Source: CAD feature listing. Evaluate the final solid. Frame: model axes, mm. A direction names the side the tool comes from. Coordinates: 2 decimals unless noted, no trailing zeros. Loops run counter-clockwise (first coordinate to the right, second up) from the corner with the lowest first, then second, coordinate; pieces in that order, holes last. Notation, with made-up numbers: M 69.5,59.5 L 87.5,59.5 A10 cw 87.5,77.5 Z; hole C -38,60 d4. An arc over 180 degrees is marked long. Write each question's results on one line, items separated by ' | '. Start each with the question number.
from build123d import *

# Parameters (mm, degrees)
BOSS_EXTRUDE2_DEPTH   = 34
SKETCH3_W             = 180.49084133
SKETCH3_H             = 138
CUT_EXTRUDE1_DEPTH    = 14
SKETCH4_R             = 11.5
SKETCH4_R_2           = 1.6
SKETCH4_R_3           = 6
CUT_EXTRUDE3_DEPTH    = 227.1769219
SKETCH5_W             = 42
SKETCH5_H             = 44
CUT_EXTRUDE4_DEPTH    = 8
M3_TAPPED_HOLE1_D     = 2.5
M3_TAPPED_HOLE1_DEPTH = 20
M3_TAPPED_HOLE1_TIP   = 0.751075774
SKETCH9_R             = 10.5
SKETCH9_R_2           = 7
CUT_EXTRUDE6_DEPTH    = 220.956813959
SKETCH10_R            = 11.5
CUT_EXTRUDE7_DEPTH    = 6
SKETCH11_R            = 13
CUT_EXTRUDE8_DEPTH    = 34
CHAMFER1_SIZE         = 6
FILLET1_R             = 10
SKETCH12_R            = 1.5
CUT_EXTRUDE9_DEPTH    = 30
SKETCH13_R            = 2.75
CUT_EXTRUDE10_DEPTH   = 3.5


with BuildPart() as part:
    # Sketch1 → Boss-Extrude2 (new body)
    with BuildSketch(Plane.XY):
        with BuildLine():
            Line((0, 0), (70, 0))
            Line((70, 0), (70, 62))
            Line((70, 62), (76, 68))
            Line((76, 68), (90, 68))
            ThreePointArc((90, 68), (97.071067812, 70.928932188), (100, 78))
            Line((100, 78), (100, 190))
            ThreePointArc((100, 190), (97.071067812, 197.071067812), (90, 200))
            Line((90, 200), (37.257365568, 200))
            ThreePointArc((37.257365568, 200), (31.383783185, 198.093270661), (27.750067173, 193.100205998))
            Line((27.750067173, 193.100205998), (-15, 62))
            Line((-15, 62), (-15, 34))
            Line((-15, 34), (0, 34))
            Line((0, 34), (0, 0))
        make_face()
    extrude(amount=BOSS_EXTRUDE2_DEPTH)

    # Sketch3 → Cut-Extrude1 (cut)
    with BuildSketch(Plane(origin=(0, 0, 0), x_dir=(-1, 0, 0), z_dir=(0, 0, -1))):
        with Locations((-9.754579335, 131)):
            Rectangle(SKETCH3_W, SKETCH3_H)
    extrude(amount=-CUT_EXTRUDE1_DEPTH, mode=Mode.SUBTRACT)

    # Sketch4 → Cut-Extrude3 (cut, through all)
    with BuildSketch(Plane.XY.offset(34)):
        with Locations((80, 134)):
            Circle(SKETCH4_R)
        with Locations((95.5, 149.5)):
            Circle(SKETCH4_R_2)
        with Locations((95.5, 118.5)):
            Circle(SKETCH4_R_2)
        with Locations((64.5, 118.5)):
            Circle(SKETCH4_R_2)
        with Locations((64.5, 149.5)):
            Circle(SKETCH4_R_2)
        with Locations((80, 174)):
            Circle(SKETCH4_R_3)
        with Locations((80, 94)):
            Circle(SKETCH4_R_3)
    extrude(amount=-CUT_EXTRUDE3_DEPTH, mode=Mode.SUBTRACT)

    # Sketch5 → Cut-Extrude4 (cut)
    with BuildSketch(Plane.XY.offset(34)):
        with Locations((79, 134)):
            Rectangle(SKETCH5_W, SKETCH5_H)
    extrude(amount=-CUT_EXTRUDE4_DEPTH, mode=Mode.SUBTRACT)

    # M3 Tapped Hole1
    with Locations(Plane(origin=(100, 0, 0), x_dir=(0, 0, -1), z_dir=(1, 0, 0))):
        with Locations((-24, 174), (-24, 94)):
            Hole(M3_TAPPED_HOLE1_D / 2, depth=M3_TAPPED_HOLE1_DEPTH)
            with Locations((0, 0, -(M3_TAPPED_HOLE1_DEPTH + M3_TAPPED_HOLE1_TIP / 2))):  # 118° drill point
                Cone(0, M3_TAPPED_HOLE1_D / 2, M3_TAPPED_HOLE1_TIP, mode=Mode.SUBTRACT)

    # Sketch9 → Cut-Extrude6 (cut, through all)
    with BuildSketch(Plane(origin=(70, 0, 0), x_dir=(0, 0, -1), z_dir=(1, 0, 0))):
        with Locations((-17, 47)):
            Circle(SKETCH9_R)
        with Locations((-17, 18)):
            Circle(SKETCH9_R_2)
    extrude(amount=-CUT_EXTRUDE6_DEPTH, mode=Mode.SUBTRACT)

    # Sketch10 → Cut-Extrude7 (cut)
    with BuildSketch(Plane.ZY):
        with Locations(Location((17, 18, 0), (0, 0, 270))):
            Circle(SKETCH10_R)
    extrude(amount=-CUT_EXTRUDE7_DEPTH, mode=Mode.SUBTRACT)

    # Sketch11 → Cut-Extrude8 (cut)
    with BuildSketch(Plane(origin=(70, 0, 0), x_dir=(0, 0, -1), z_dir=(1, 0, 0))):
        with Locations((-17, 18)):
            Circle(SKETCH11_R)
    extrude(amount=-CUT_EXTRUDE8_DEPTH, mode=Mode.SUBTRACT)

    # Chamfer1
    chamfer1_edges = [part.edges().sort_by_distance(p)[0] for p in [
        (27.5, 62, 0),
        (27.5, 62, 14),
    ]]
    chamfer(chamfer1_edges, length=CHAMFER1_SIZE)

    # Fillet1
    fillet1_edges = [part.edges().sort_by_distance(p)[0] for p in [
        (35, 0, 0),
        (35, 0, 34),
    ]]
    fillet(fillet1_edges, radius=FILLET1_R)

    # Sketch12 → Cut-Extrude9 (cut)
    with BuildSketch(Plane.ZY.offset(-6)):
        with Locations((17, 26)):
            Circle(SKETCH12_R)
        with Locations((25, 18)):
            Circle(SKETCH12_R)
        with Locations((17, 10)):
            Circle(SKETCH12_R)
        with Locations((9, 18)):
            Circle(SKETCH12_R)
    extrude(amount=-CUT_EXTRUDE9_DEPTH, mode=Mode.SUBTRACT)

    # Sketch13 → Cut-Extrude10 (cut)
    with BuildSketch(Plane(origin=(0, 0, 14), x_dir=(-1, 0, 0), z_dir=(0, 0, -1))):
        with Locations((-95.5, 149.5)):
            Circle(SKETCH13_R)
        with Locations((-64.5, 149.5)):
            Circle(SKETCH13_R)
        with Locations((-64.5, 118.5)):
            Circle(SKETCH13_R)
        with Locations((-95.5, 118.5)):
            Circle(SKETCH13_R)
    extrude(amount=-CUT_EXTRUDE10_DEPTH, mode=Mode.SUBTRACT)


solid = part.part
Item 1: Cut plane A-A (x = 3). Output: boundary loops of the cut face in (y, z), then the cut area to 3 significant figures.
Item 2: Access query for faces 5 (the cylindrical face through (97.682, 116.827, 15.726)), 6 (the flat face through (70, 31, 21)), 7 (the flat face through (57, 135, 14)), 8 (the flat face through (6, 13, 22.3)), 9 (the flat face through (69, 139, 26)). Directions: +Z, -Z, +X, -X, +Y, -Y. A direction counts if a zero-diameter tool reaches every point of the face in a straight line with its end or side. Return the directions, or none.
Item 3: Cut plane C-C (x = 55.5). Output: boundary loops of the cut face in (y, z), then the cut area to 3 significant figures.
Item 4: First-contact query: pin 1 Ø4.5 at (x, y) = (96.5, 119) entering from -Z; pin 2 Ø4 at (x, y) = (67, 129) entering from +Z; pin 3 Ø4 at (x, y) = (64.5, 118.5) entering from -Z; pin 4 Ø6 at (y, z) = (87.5, 11.5) entering from +X. Flat tips, straight axial feed; report the tip coordinate or a pass-through.
Item 5: Line query: probe 1 along Y at (x, z) = (44, 17); probe 2 along Z at (x, y) = (25.5, 26); probe 3 along Y at (x, z) = (50.5, 23). Output: solid intervals per line, ascending.
Item 6: Cut plane B-B (z = 20.5). Count the separate pieces of the cut face and the enclosed holes in it, then the cut area to 3 significant figures.
Item 7: Cut plane D-D (y = 183). Output: boundary loops of the cut face in (x, z), then the cut area to 3 significant figures.
Item 8: Mould query, pull axis X, two halves, no side actions, for faces 1 (the cylindrical face through (35.49, 2.85, 3.01)), 2 (the flat face through (0, 17, 5)), 3 (the flat face through (94, 148, 17.5)), 4 (the flat face through (63, 148, 17.5)). Classes: +X half, -X half, draft (parallel to the pull), parting line (faces both ways), or undercut.
Response values:
1) outline: M 0,10 A10 ccw 10,0 L 56,0 L 62,6 L 62,8 L 68,14 L 117.2,14 L 117.2,34 L 10,34 A10 ccw 0,24 Z; hole C 18,17 d23; hole C 47,17 d21 | area: 2,410 mm2
2) face 5: -Z | face 6: +Z, -Z, +X, -Y | face 7: -Z, +X, -X, +Y | face 8: -X | face 9: +Z, +X
3) outline: M 0,10 A10 ccw 10,0 L 56,0 L 62,6 L 62,8 L 68,14 L 200,14 L 200,34 L 10,34 A10 ccw 0,24 Z; hole C 18,17 d26; hole C 47,17 d21 | area: 3,950 mm2
4) pin 1: stops at z = 14 | pin 2: stops at z = 26 | pin 3: stops at z = 17.5 | pin 4: stops at x = 100
5) probe 1: y = 0 to 5, 31 to 36.5, 57.5 to 200 | probe 2: z = 0 to 15.5, 18.5 to 34 | probe 3: y = 0 to 6.47, 29.53 to 38.38, 55.62 to 200
6) separate pieces: 3 | enclosed holes: 7 | area: 13,600 mm2
7) outline: M 24.46,14 L 100,14 L 100,34 L 24.46,34 Z | area: 1,510 mm2
8) face 1: draft | face 2: -X half | face 3: undercut | face 4: undercut
